Can you work these out from the drawing? Everything is in mm from the part's minimum corner. Give positions to 0.01 mm unless a question says otherwise; leave off trailing zeros. Loops run counter-clockwise (first coordinate to the right, second up) from the corner with the lowest first, then second, coordinate; pieces in that order, holes last.
Q1. If we section it at C-C (z = 76): Please give me the cut outline in (x, y), plus the area to 3 significant figures.
Q2. Will these pins go through, and if not, where does the flat tip stop? P1, Ø15, axis at y = 6, z = 141.5, coming from the -X side; P2, Ø15, axis at y = 11, z = 142.5, coming from the +X side; P3, Ø5, axis at x = 77, z = 47.5, coming from the +Y side.
Q3. If we section it at A-A (y = 11.5): Please give me the cut outline in (x, z), plus the area to 3 significant figures.
Q4. If we section it at B-B (x = 32): Please give me the cut outline in (y, z).
Q5. We'd pull the mould along X, two halves only. Please class the marked faces 1, 2 and 3: +X half, -X half, draft (parallel to the pull), parting line (faces both ways), or undercut.
Q6. I need wall thicknesses on line 1 (Z direction, x = 182.5, y = 10); line 2 (Y direction, x = 84.5, z = 89) (1 decimal); line 3 (Y direction, x = 166, z = 23.5) (1 decimal). Which ranges of each line are inside material? Lowest first, please.
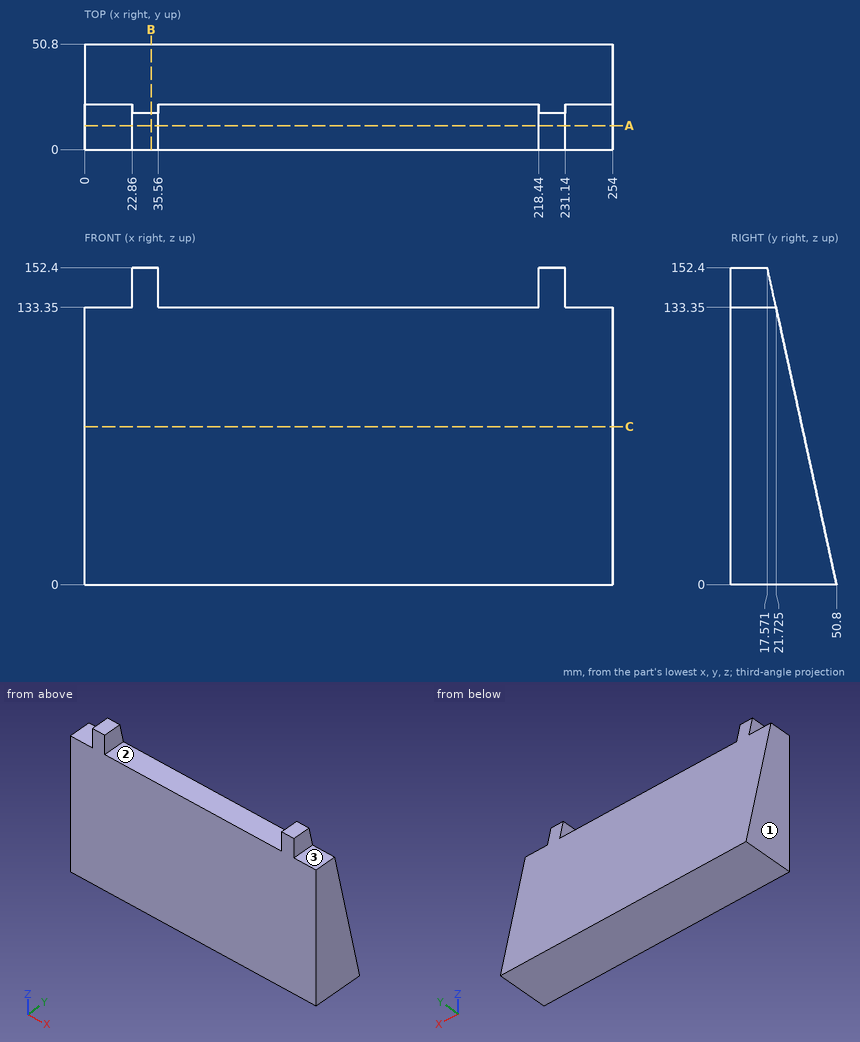
Check sheet entries:
1. outline: (0, 0) - (254, 0) - (254, 34.23) - (0, 34.23) - close
1. area: 8,690 mm2
2. P1: stops at x = 22.86
2. P2: stops at x = 231.14
2. P3: stops at y = 40.99
3. outline: (0, 0) - (254, 0) - (254, 133.35) - (231.14, 133.35) - (231.14, 152.4) - (218.44, 152.4) - (218.44, 133.35) - (35.56, 133.35) - (35.56, 152.4) - (22.86, 152.4) - (22.86, 133.35) - (0, 133.35) - close
3. area: 34,400 mm2
4. outline: (0, 0) - (50.8, 0) - (17.57, 152.4) - (0, 152.4) - close
5. face 1: -X half
5. face 2: undercut
5. face 3: draft
6. line 1: z = 0 to 133.35
6. line 2: y = 0 to 31.4
6. line 3: y = 0 to 45.7
